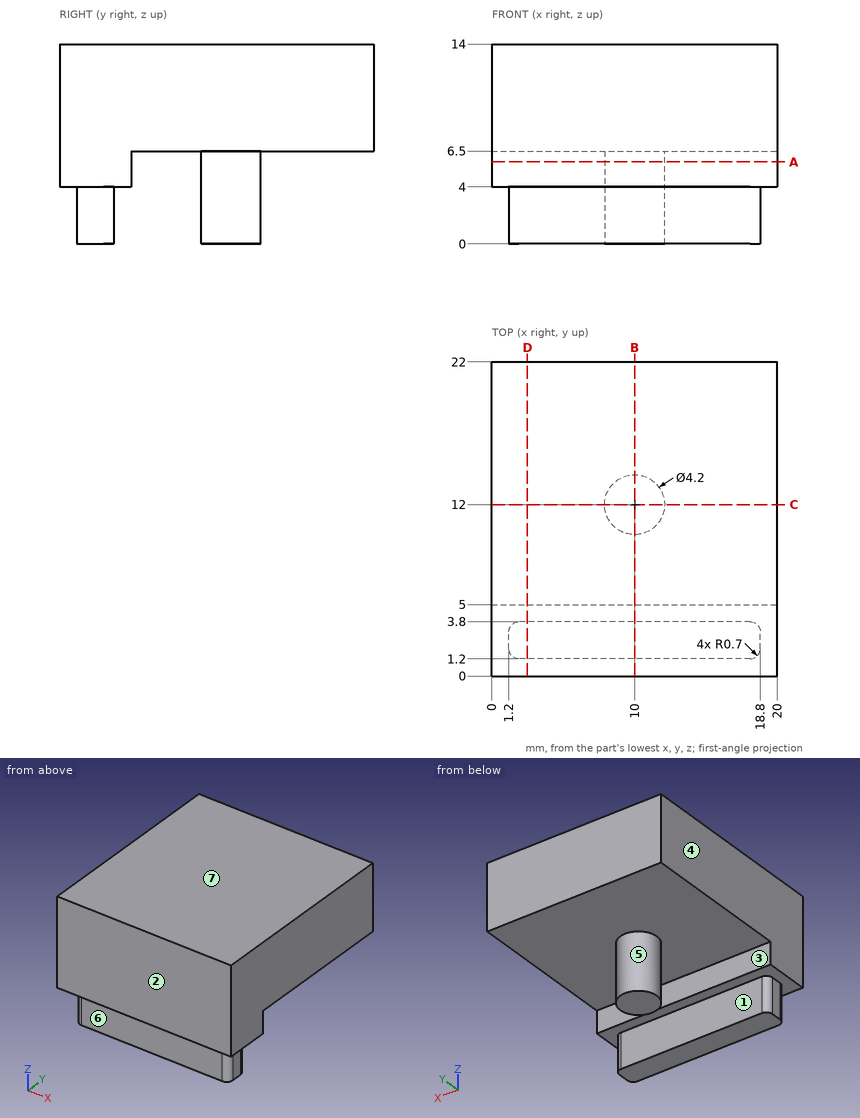
Here's the drawing with two shaded views (mm, measured from the low corner). I have some questions. A direction names the side the tool comes from. Give positions to 0.01 mm unless a question says otherwise; leave off trailing zeros. Loops run counter-clockwise (first coordinate to the right, second up) from the corner with the lowest first, then second, coordinate; pieces in that order, holes last. Notation, with made-up numbers: M -29,38.25 L -16,38.25 A3 cw -16,43.25 Z; hole C 60,65.5 d8. An arc over 180 degrees is marked long. One line per item, written item: value. Start each with the question number.
1) If we section it at B-B, the plane x = 10: Write out the boundary of the cut face in (y, z), and give its area (3 significant figures).
2) If we section it at C-C, the plane y = 12: Write out the boundary of the cut face in (x, z), and give its area (3 significant figures).
3) On a 3-axis mill with a long thin cutter (end or side, diameter ignored), from which of +Z, -Z, +X, -X, +Y, -Y can I reach the whole of each face in a straight line? I mean the marked faces 5, 6 and 7. Say none if no direction works.
4) If we section it at D-D, the plane x = 2.5: Write out the boundary of the cut face in (y, z), and give its area (3 significant figures).
5) Thinking about a two-plate mould opening in Y: for the marked faces 1, 2, 3 and 4, which applies, +Y half, -Y half, draft (parallel to the pull), parting line (faces both ways), or undercut?
6) If we section it at A-A, the plane z = 5.75: Write out the boundary of the cut face in (x, y).
7) I'm going to push flat-ended pins straight in: pin 1 (1.3 mm diameter, centred on y = 2.5, z = 1, fed in from +X); pin 2 (1.3 mm diameter, centred on y = 2.5, z = 1, fed in from -X); pin 3 (1 mm diameter, centred on y = 19.5, z = 5, fed in from -X); pin 4 (2 mm diameter, centred on x = 12, z = 2, fed in from +Y). Where does each tip first touch, or does it pass through?
8) If I drill on line 1 (Z direction, x = 6.5, y = 5.25); line 2 (Y direction, x = 17.5, z = 2); line 3 (Y direction, x = 16.75, z = 6), over which ranges is the centre line in solid material (lowest first)? Write a range as [from, to].
Completed:
1. outline: M 0,4 L 1.2,4 L 1.2,0 L 3.8,0 L 3.8,4 L 5,4 L 5,6.5 L 9.9,6.5 L 9.9,0 L 14.1,0 L 14.1,6.5 L 22,6.5 L 22,14 L 0,14 Z
1. area: 215 mm^2
2. outline: M 0,6.5 L 7.9,6.5 L 7.9,0 L 12.1,0 L 12.1,6.5 L 20,6.5 L 20,14 L 0,14 Z
2. area: 177 mm^2
3. face 5: -Z
3. face 6: -Z, +X, -X, -Y
3. face 7: +Z, +X, -X, +Y, -Y
4. outline: M 0,4 L 1.2,4 L 1.2,0 L 3.8,0 L 3.8,4 L 5,4 L 5,6.5 L 22,6.5 L 22,14 L 0,14 Z
4. area: 188 mm^2
5. face 1: undercut
5. face 2: -Y half
5. face 3: undercut
5. face 4: draft
6. outline: M 0,0 L 20,0 L 20,5 L 0,5 Z; C 10,12 d4.2
7. pin 1: stops at x = 18.8
7. pin 2: stops at x = 1.2
7. pin 3: passes through
7. pin 4: stops at y = 13.85
8. line 1: z = [6.5, 14]
8. line 2: y = [1.2, 3.8]
8. line 3: y = [0, 5]
